from build123d import *

# Parameters (mm, degrees)
SKETCH1_R           = 11025
BOSS_EXTRUDE1_DEPTH = 5000
BOSS_EXTRUDE2_DEPTH = 8000
SKETCH4_R           = 3000
CUT_EXTRUDE2_DEPTH  = 3000
SKETCH5_R           = 1500
CUT_EXTRUDE3_DEPTH  = 3000
SKETCH6_R           = 3000
CUT_EXTRUDE4_DEPTH  = 3000
SKETCH3_R           = 2900
CUT_EXTRUDE1_DEPTH  = 12018
SCALE6_SCALE        = 0.001


with BuildPart() as part:
    # Sketch1 → Boss-Extrude1 (new body)
    with BuildSketch(Plane.XY):
        Polygon((-21150, 17212.99935917), (-17091.781053823, 21271.218305346), (17091.781053823, 21271.218305346), (21150, 17212.99935917), (21150, -16970.562748477), (17091.781053823, -21028.781694654), (-17091.781053823, -21028.781694654), (-21150, -16970.562748477), align=None)
        with Locations((0, 121.218305346)):
            Circle(SKETCH1_R, mode=Mode.SUBTRACT)
    extrude(amount=BOSS_EXTRUDE1_DEPTH)

    # Sketch2 → Boss-Extrude2 (add)
    with BuildSketch(Plane.XY.offset(5000)):
        Polygon((0, -11028.781694654), (4500, -11028.781694654), (4500, -21028.781694654), (-4500, -21028.781694654), (-4500, -11028.781694654), align=None)
    extrude(amount=BOSS_EXTRUDE2_DEPTH)

    # Sketch4 → Cut-Extrude2 (cut)
    with BuildSketch(Plane.XY.offset(5000)):
        with Locations((-15500, 15500)):
            Circle(SKETCH4_R)
        with Locations((15500, 15500)):
            Circle(SKETCH4_R)
        with Locations((15500, -15500)):
            Circle(SKETCH4_R)
        with Locations((-15500, -15500)):
            Circle(SKETCH4_R)
    extrude(amount=-CUT_EXTRUDE2_DEPTH, mode=Mode.SUBTRACT)

    # Sketch5 → Cut-Extrude3 (cut)
    with BuildSketch(Plane.XY.offset(2000)):
        with Locations((-15500, 15500)):
            Circle(SKETCH5_R)
        with Locations((15500, -15500)):
            Circle(SKETCH5_R)
    extrude(amount=-CUT_EXTRUDE3_DEPTH, mode=Mode.SUBTRACT)

    # Sketch6 → Cut-Extrude4 (cut)
    with BuildSketch(Plane.XY.offset(2000)):
        with Locations((15500, 15500)):
            Circle(SKETCH6_R)
        with Locations((-15500, -15500)):
            Circle(SKETCH6_R)
    extrude(amount=-CUT_EXTRUDE4_DEPTH, mode=Mode.SUBTRACT)

    # Sketch3 → Cut-Extrude1 (cut)
    with BuildSketch(Plane.XZ.offset(21028.781694654)):
        with Locations(Location((0, 9000, 0), (0, 0, 270))):
            Circle(SKETCH3_R)
    extrude(amount=-CUT_EXTRUDE1_DEPTH, mode=Mode.SUBTRACT)


with BuildPart() as part_1:
    # Scale6: scaled about (0, -945.258123271, 2914.075668663)
    add(part.part.scale(SCALE6_SCALE).moved(Location((0, -944.312865148, 2911.161592994))))


solid = part_1.part
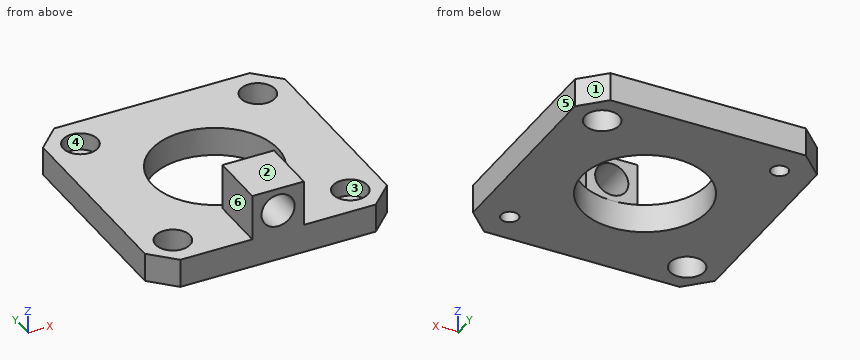
Build history of the part. All positions in model axes, mm. Face numbers are marked on the shaded views. A direction names the side the tool comes from. Coordinates: 2 decimals unless noted, no trailing zeros. Write each loop counter-clockwise with the first axis right and the second up, starting at its lowest first coordinate (ties: lowest second). Pieces come first, ordered by that corner, then holes.
(1) 3-axis set-ups, long thin cutter, end or side, ignore diameter. For the marked faces 4, 5 and 6: which of +Z, -Z, +X, -X, +Y, -Y reach the whole face in a straight line?
(2) Pin check, flat tips, straight feed: pin 1 Ø4 at (y, z) = (-958, 2918.5) entering from +X; pin 2 Ø2.5 at (y, z) = (-961.5, 2920.5) entering from -X; pin 3 Ø12 at (x, y) = (8.5, -943) entering from +Z. Stop position of each tip, or through.
(3) Drill centre lines: line 1 (Y direction, x = 15.5, z = 2914.9); line 2 (Y direction, x = -15.5, z = 2912.5); line 3 (Y direction, x = 0, z = 2913.75). Where is each one in solid material? Low to high.
(4) Mould opens along X. For the marked faces 1, 2 and 3 say: pulls with the +X half, pulls with the -X half, needs draft (parallel to the pull), parting line crosses it, or undercut.
(5) Cut at B-B on y = -959. List the corners of the cut face in (x, z), and give its area (3 significant figures).
(6) Cut at D-D on x = -10. List the corners of the cut face in (y, z).
(7) Cut at A-A on x = 0. List the corners of the cut face in (y, z).
(8) Cut at C-C on z = 2912.5. List the corners of the cut face in (x, y) (3 decimals).
Working result:
1. face 4: +Z
1. face 5: +Z, -Z, +X, +Y, -Y
1. face 6: +Z, -X, +Y, -Y
2. pin 1: stops at x = 4.5
2. pin 2: stops at x = -4.5
2. pin 3: stops at z = 2916.16
3. line 1: y = -965.34 to -962.81, -956.81 to -931.81, -925.81 to -923.04
3. line 2: y = -965.34 to -962.81, -956.81 to -930.31, -927.31 to -923.04
3. line 3: y = -965.34 to -955.22, -933.17 to -923.04
4. face 1: pulls with the +X half
4. face 2: needs draft
4. face 3: undercut
5. outline: (-21.15, 2911.16) - (-18.39, 2911.16) - (-18.39, 2916.16) - (-21.15, 2916.16) - close; (-12.61, 2911.16) - (14.24, 2911.16) - (14.24, 2913.16) - (12.61, 2913.16) - (12.61, 2916.16) - (4.5, 2916.16) - (4.5, 2924.16) - (-4.5, 2924.16) - (-4.5, 2916.16) - (-12.61, 2916.16) - close; (16.76, 2911.16) - (21.15, 2911.16) - (21.15, 2916.16) - (18.39, 2916.16) - (18.39, 2913.16) - (16.76, 2913.16) - close; hole circle Ø5.8 at (0, 2920.16)
5. area: 206 mm2
6. outline: (-965.34, 2911.16) - (-948.83, 2911.16) - (-948.83, 2916.16) - (-965.34, 2916.16) - close; (-939.55, 2911.16) - (-923.04, 2911.16) - (-923.04, 2916.16) - (-939.55, 2916.16) - close
7. outline: (-965.34, 2911.16) - (-955.22, 2911.16) - (-955.22, 2916.16) - (-955.34, 2916.16) - (-955.34, 2917.26) - (-965.34, 2917.26) - close; (-965.34, 2923.06) - (-955.34, 2923.06) - (-955.34, 2924.16) - (-965.34, 2924.16) - close; (-933.17, 2911.16) - (-923.04, 2911.16) - (-923.04, 2916.16) - (-933.17, 2916.16) - close
8. outline: (-21.15, -961.283) - (-17.092, -965.342) - (17.092, -965.342) - (21.15, -961.283) - (21.15, -927.1) - (17.092, -923.042) - (-17.092, -923.042) - (-21.15, -927.1) - close; hole circle Ø6 at (-15.5, -959.813); hole circle Ø3 at (-15.5, -928.813); hole circle Ø22.05 at (0, -944.192); hole circle Ø6 at (15.5, -928.813); hole circle Ø3 at (15.5, -959.813)
